Check sheet for the modelled part. Datum: model origin and axes. Units: mm. Face numbers are marked on the shaded views. A direction names the side the tool comes from. Coordinates: 2 decimals unless noted, no trailing zeros. Loops run counter-clockwise (first coordinate to the right, second up) from the corner with the lowest first, then second, coordinate; pieces in that order, holes last. Notation, with made-up numbers: (50, -29.5) -> (88, -29.5) arc R17 cw to (88, -1.5) -> close; hole circle Ø9 at (55, -16.75). An arc over 180 degrees is marked (long way). Use one line per item in the form item = value.
from build123d import *

# Parameters (mm, degrees)
F0_R     = 2.5
F1_DEPTH = 15
F2_R     = 5
F4_DEPTH = 25


with BuildPart() as f1:
    # F0 (on Front) → F1 (new body)
    with BuildSketch(Plane.XZ):
        Polygon((5, 45), (-5, 45), (-5, 5), (-45, 5), (-45, -5), (5, -5), align=None)
        Circle(F0_R, mode=Mode.SUBTRACT)
    extrude(amount=F1_DEPTH)

    # F2
    f2_edges = [f1.edges().sort_by_distance(p)[0] for p in [
        (-5, -7.5, 5),
    ]]
    fillet(f2_edges, radius=F2_R)

    # F3 (on Front) → F4 (cut)
    with BuildSketch(Plane.XZ):
        with BuildLine():
            ThreePointArc((-10, 5), (-8.842421, 4.715854), (-7.947978, 3.928008))
            ThreePointArc((-7.947978, 3.928008), (-3.535534, 3.535534), (-3.928008, 7.947978))
            ThreePointArc((-3.928008, 7.947978), (-4.715854, 8.842421), (-5, 10))
            ThreePointArc((-5, 10), (-6.464466, 6.464466), (-10, 5))
        make_face()
    extrude(amount=F4_DEPTH, mode=Mode.SUBTRACT)


solid = f1.part
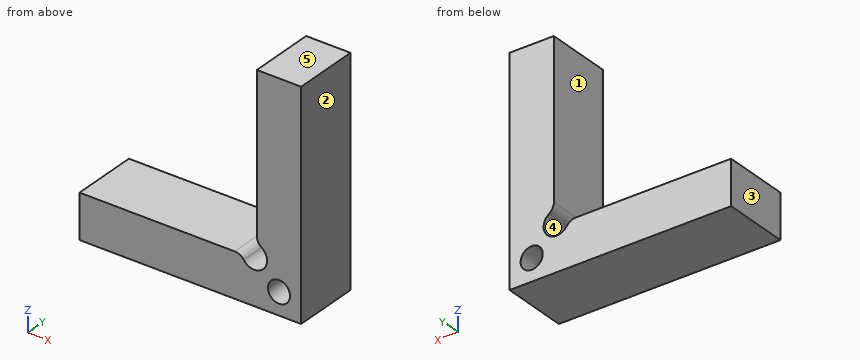
(1) Section check B-B, the plane z = 0. Record the boundary of the cut face in (x, y), plus the area to 3 significant figures.
Established:
outline = (-45, -15) -> (-2.5, -15) -> (-2.5, 0) -> (-45, 0) -> close; (2.5, -15) -> (5, -15) -> (5, 0) -> (2.5, 0) -> close
area = 675 mm²
(2) Mould release check, pull along X, two halves, no side actions. Record for the marked faces 3, 4 and 5: +X half, -X half, draft (parallel to the pull), parting line (faces both ways), or undercut.
Established:
face_3 = -X half
face_4 = undercut
face_5 = draft
(3) Scan lines: line 1 along Z through (x, y) = (0, -4); line 2 along Z through (x, y) = (-24.5, -1). Record each from-to range of solid material in increasing order.
Established:
line_1 = -5 to -2.5, 2.5 to 45
line_2 = -5 to 5
(4) Go/stop test with flat-tipped pins: P1, Ø4.5, axis at x = 0, z = 0, coming from the +Y side (3 decimals); P2, Ø1, axis at x = -35, y = -13.5, coming from the +Z side; P3, Ø5, axis at y = -5, z = 30.5, coming from the -X side. Record where each tip stops, or that it passes through.
Established:
P1 = through
P2 = 5
P3 = -5
(5) Tool access check on the marked faces 1 and 2. Record the directions out of +Z, -Z, +X, -X, +Y, -Y that give a thin tool (end or side, any length) a straight path to the whole face; none if there is none.
Established:
face_1 = +Z, -X, +Y, -Y
face_2 = +Z, -Z, +X, +Y, -Y
(6) Section check C-C, the plane y = -12.25. Record the boundary of the cut face in (x, z).
Established:
outline = (-45, -5) -> (5, -5) -> (5, 45) -> (-5, 45) -> (-5, 10) arc R2.5 ccw to (-3.93, 7.95) arc R2.89 cw (long way) to (-7.95, 3.93) arc R2.5 ccw to (-10, 5) -> (-45, 5) -> close; hole circle Ø5 at (0, 0)
(7) Section check A-A, the plane x = 0. Record the boundary of the cut face in (y, z), plus the area to 3 significant figures.
Established:
outline = (-15, -5) -> (0, -5) -> (0, -2.5) -> (-15, -2.5) -> close; (-15, 2.5) -> (0, 2.5) -> (0, 45) -> (-15, 45) -> close
area = 675 mm²
(8) Section check D-D, the plane z = 33.5. Record the boundary of the cut face in (x, y), plus the area to 3 significant figures.
Established:
outline = (-5, -15) -> (5, -15) -> (5, 0) -> (-5, 0) -> close
area = 150 mm²
